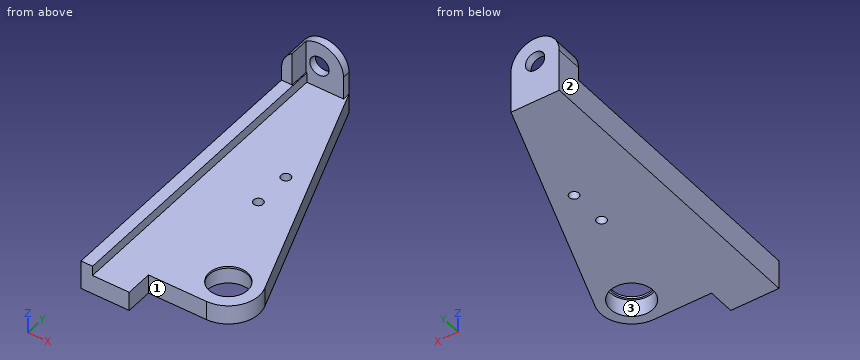
Autodesk Inventor part; units mm, degrees
ref_plane "YZ Plane" through (0, 0, 0) normal (1, 0, 0) x (0, 1, 0)
ref_plane "XZ Plane" through (0, 0, 0) normal (0, 1, 0) x (-1, 0, 0)
ref_plane "XY Plane" through (0, 0, 0) normal (0, 0, 1) x (1, 0, 0)
sketch "Sketch1" plane through (0, 0, 0) normal (0, 0, 1) x (1, 0, 0)
  circle A0 centre (0, 0) radius 11
  line L0 (0, 0) -> (-30, 0) construction
  line L1 (0, 16) -> (-30, 16)
  line L2 (-30, -16) -> (0, -16)
  arc A1 (0, -16) -> (0, 16) centre (0, 0) ccw
  arc A2 (-30, 16) -> (-30, -16) centre (-30, 0) ccw construction
  line L3 (-30, 16) -> (-30, -16)
  line L4 (-30, 130) -> (-55, 130)
  line L5 (-55, 130) -> (-55, -130)
  line L6 (-55, -130) -> (-30, -130)
  line L7 (-30, -130) -> (-30, 130)
  point P0 (-15, 0)
  point P1 (-30, 0)
  dimension "d0" = 22
  dimension "d1" = 5
  dimension "d2" = 30
  dimension "d3" = 260
  dimension "d4" = 25
extrude "Extrusion1" add sketch "Sketch1" along normal blind 10
sketch "Sketch2" plane through (-55, 130, 0) normal (0, 1, 0) x (1, 0, 0)
  line L0 (25, -10) -> (0, -10) construction
  line L1 (12.5, -10) -> (12.5, -22) construction
  circle A0 centre (12.5, -22) radius 5
  line L2 (12.5, -10) -> (12.5, -22) construction
  line L3 (25, -10) -> (25, -22)
  line L4 (0, -22) -> (0, -10)
  arc A1 (25, -10) -> (0, -10) centre (12.5, -10) ccw construction
  arc A2 (0, -22) -> (25, -22) centre (12.5, -22) ccw
  line L5 (0, -10) -> (25, -10)
  point P0 (55, 0)
  point P1 (12.5, -16)
  dimension "d7" = 10
  dimension "d8" = 12
extrude "Extrusion2" add sketch "Sketch2" against normal blind 4
sketch "Sketch3" plane through (0, 0, 10) normal (0, 0, 1) x (1, 0, 0)
  line L0 (-55, 130) -> (-55, -130)
  line L1 (-55, -130) -> (-30, -130)
  line L2 (-55, -130) -> (-30, -130)
  line L3 (-30, -130) -> (-30, -30)
  line L4 (-30, -30) -> (-55, -30)
  line L5 (-55, -30) -> (-55, -130)
  point P0 (0, 0)
  dimension "d11" = 100
extrude "Extrusion3" cut sketch "Sketch3" against normal through all
sketch "Sketch4" plane through (0, 0, 10) normal (0, 0, 1) x (1, 0, 0)
  line L0 (-55, -30) -> (-49, -30)
  line L1 (-49, -30) -> (-49, 126)
  line L2 (-49, 126) -> (-55, 126)
  line L3 (-55, 126) -> (-55, -30)
  line L4 (-55, 126) -> (-30, 126)
  line L5 (-49, 3) -> (-49, -97) construction
  point P0 (0, 0)
  dimension "d18" = 6
extrude "Extrusion4" add sketch "Sketch4" along normal blind 5.1
sketch "Sketch5" plane through (-55, 126, 0) normal (0, -1, 0) x (1, 0, 0)
  line L0 (5.5, 23.8249) -> (5.5, 20.1751) construction
  line L1 (0, 15.1) -> (6, 15.1)
  line L2 (0, 15.1) -> (5.5, 15.1)
  line L3 (5.5, 15.1) -> (5.5, 22)
  line L4 (5.5, 22) -> (0, 22)
  line L5 (0, 22) -> (0, 15.1)
  line L6 (5.5, 22) -> (5.5, 32.3562)
  arc A0 (25, 22) -> (0, 22) centre (12.5, 22) ccw
  arc A1 (5.5, 32.3562) -> (0, 22) centre (12.5, 22) ccw
  line L7 (5.5, 22) -> (0, 22)
  point P0 (55, 0)
extrude "Extrusion5" add sketch "Sketch5" along normal blind 10
sketch "Sketch6" plane through (0, 0, 0) normal (0, 0, -1) x (-1, 0, 0)
  line L0 (30, 130) -> (-15.0463, 5.4414)
  arc A0 (0, 16) -> (0, -16) centre (0, 0) ccw
  arc A1 (0, 16) -> (-15.0463, 5.4414) centre (0, 0) ccw
  line L1 (0, 16) -> (30, 16)
  line L2 (0, 16) -> (30, 16)
  line L3 (30, 16) -> (30, 130)
  line L4 (30, 16) -> (30, 130)
extrude "Extrusion6" add sketch "Sketch6" against normal up to surface (10 mm away)
sketch "Sketch7" plane through (0, 0, 10) normal (0, 0, 1) x (1, 0, 0)
  line L0 (-20, 50) -> (-20, 70) construction
  circle A0 centre (-20, 50) radius 2.5
  circle A1 centre (-20, 70) radius 2.5
  line L1 (-55, 116) -> (-55, -30)
  line L2 (-30, 130) -> (-55, 130)
  point P0 (0, 0)
  dimension "d21" = 5
  dimension "d22" = 20
  dimension "d23" = 35
  dimension "d24" = 80
extrude "Extrusion7" cut sketch "Sketch7" against normal through all
sketch "Sketch8" plane through (0, 0, 10) normal (0, 0, 1) x (1, 0, 0)
  circle A0 centre (0, 0) radius 11
  circle A1 centre (0, 0) radius 10
  dimension "d27" = 1
extrude "Extrusion8" add sketch "Sketch8" against normal blind 1
properties part number "frame"
Geometry: final body of the model. Coordinates: model frame, mm. Face numbers are marked on the shaded views. Coordinates: 2 decimals unless noted, no trailing zeros. Order: outer loops, then holes, each group sorted by start corner. A loop starts at its lowest first (then second) coordinate and runs counter-clockwise, first axis right, second up.
Item 1: Section query D-D (z = 7). Output: boundary loops of the cut face in (x, y), then the cut area to 3 significant figures.
Answer:
outline: (-55, -30) - (-30, -30) - (-30, -16) - (0, -16) arc R16 ccw to (15.05, 5.44) - (-30, 130) - (-55, 130) - close; hole circle Ø5 at (-20, 50); hole circle Ø5 at (-20, 70); hole circle Ø22 at (0, 0)
area: 7,320 mm2
Item 2: Section query B-B (y = 0). Output: boundary loops of the cut face in (x, z).
Answer:
outline: (-55, 0) - (-11, 0) - (-11, 9) - (-10, 9) - (-10, 10) - (-49, 10) - (-49, 15.1) - (-55, 15.1) - close; (10, 9) - (11, 9) - (11, 0) - (16, 0) - (16, 10) - (10, 10) - close
Item 3: Section query C-C (z = 20). Output: boundary loops of the cut face in (x, y), then the cut area to 3 significant figures.
Answer:
outline: (-55, 116) - (-49.5, 116) - (-49.5, 126) - (-47.08, 126) - (-47.08, 130) - (-55, 130) - close; (-37.92, 126) - (-30, 126) - (-30, 130) - (-37.92, 130) - close
area: 118 mm2
Item 4: Draft query along Y for the marked faces 1, 2 and 3. Return one class per face: released by +Y, released by -Y, zero draft, split by the parting line, or undercut.
Answer:
face 1: released by -Y
face 2: zero draft
face 3: undercut
Item 5: Material intervals for line 1 along Z through (x, y) = (-49.5, -18); line 2 along Z through (x, y) = (-47.5, 111); line 3 along X through (y, z) = (79.5, 13), sorted ascending.
Answer:
line 1: z = 0 to 15.1
line 2: z = 0 to 10
line 3: x = -55 to -49
Item 6: Section query A-A (x = -42.5). Output: boundary loops of the cut face in (y, z).
Answer:
outline: (-30, 0) - (130, 0) - (130, 17) - (126, 17) - (126, 10) - (-30, 10) - close; (126, 27) - (130, 27) - (130, 34.5) - (126, 34.5) - close
Item 7: Contact query for flat-ended pins moving along their axis: P1, Ø1.7, axis at x = -53, z = 23.5, coming from the -Y side; P2, Ø4.5, axis at y = 128.5, z = 13.5, coming from the +X side; P3, Ø8, axis at x = -20, y = 50, coming from the +Z side. Output: stop coordinate, or through.
Answer:
P1: stops at y = 116
P2: stops at x = -30
P3: stops at z = 10
